Read the model definition and answer for the solid it produces. Units are mm, in the model's axes. A direction names the side the tool comes from. Give positions to 0.01 mm unless a question says otherwise; leave off trailing zeros. Order: outer loops, then holes, each group sorted by start corner. A loop starts at its lowest first (then second) coordinate and runs counter-clockwise, first axis right, second up. Notation, with made-up numbers: M -40,60.25 L -10,60.25 A13 ccw -10,67.25 Z; hole C -14,-29.5 d6. An arc over 180 degrees is marked long. Write item = value, one per line. Start each with the question number.
Autodesk Inventor part; units mm, degrees
ref_plane "YZ Plane" through (0, 0, 0) normal (1, 0, 0) x (0, 1, 0)
ref_plane "XZ Plane" through (0, 0, 0) normal (0, 1, 0) x (-1, 0, 0)
ref_plane "XY Plane" through (0, 0, 0) normal (0, 0, 1) x (1, 0, 0)
sketch "Sketch1" plane through (0, 0, 0) normal (0, 0, 1) x (1, 0, 0)
  circle A0 centre (0, 0) radius 35
  dimension "d0" = 70
extrude "Extrusion1" add sketch "Sketch1" along normal blind 50
sketch "Sketch4" plane through (0, 0, 50) normal (0, 0, 1) x (1, 0, 0)
  circle A0 centre (30, 0) radius 1.5
  dimension "d104" = 3
sketch "Sketch6" plane through (0, 0, 50) normal (0, 0, 1) x (1, 0, 0)
  circle A0 centre (-30, 0) radius 1.5
  point P0 (0, 0)
  dimension "d105" = 3
sketch "Sketch11" plane through (0, 0, 0) normal (0, 0, -1) x (-1, 0, 0)
  line L0 (13.8079, 12.25) -> (-13.8079, 12.25)
  line L1 (-18.25, 8.6641) -> (-18.25, -8.6641)
  line L2 (-13.8079, -12.25) -> (13.8079, -12.25)
  line L3 (18.25, -8.6641) -> (18.25, 8.6641)
  line L4 (17.3393, 10.3414) -> (14.8972, 11.9273)
  line L5 (17.3393, -10.3414) -> (14.8972, -11.9273)
  line L6 (-17.3393, 10.3414) -> (-14.8972, 11.9273)
  line L7 (-17.3393, -10.3414) -> (-14.8972, -11.9273)
  arc A0 (18.25, 8.6641) -> (17.3393, 10.3414) centre (16.25, 8.6641) ccw
  arc A1 (14.8972, 11.9273) -> (13.8079, 12.25) centre (13.8079, 10.25) ccw
  arc A2 (17.3393, -10.3414) -> (18.25, -8.6641) centre (16.25, -8.6641) ccw
  arc A3 (13.8079, -12.25) -> (14.8972, -11.9273) centre (13.8079, -10.25) ccw
  arc A4 (-14.8972, -11.9273) -> (-13.8079, -12.25) centre (-13.8079, -10.25) ccw
  arc A5 (-18.25, -8.6641) -> (-17.3393, -10.3414) centre (-16.25, -8.6641) ccw
  arc A6 (-17.3393, 10.3414) -> (-18.25, 8.6641) centre (-16.25, 8.6641) ccw
  arc A7 (-13.8079, 12.25) -> (-14.8972, 11.9273) centre (-13.8079, 10.25) ccw
  point P0 (18.25, 12.25)
  point P1 (-18.25, -12.25)
  point P2 (-18.25, 12.25)
  point P3 (18.25, -12.25)
  point P4 (18.25, 9.75)
  point P5 (18.25, -9.75)
  point P6 (-18.25, 9.75)
  point P7 (-18.25, -9.75)
  dimension "d73" = 36.5
  dimension "d74" = 24.5
  dimension "d75" = 2.5
  dimension "d76" = 57
  dimension "d77" = 2.5
  dimension "d78" = 57
  dimension "d79" = 2.5
  dimension "d80" = 57
  dimension "d81" = 2.5
  dimension "d82" = 57
  dimension "d83" = 2
extrude "Extrusion2" cut sketch "Sketch11" against normal blind 27.5
sketch "Sketch12" plane through (0, 0, 50) normal (0, 0, 1) x (1, 0, 0)
  line L0 (0, 0) -> (30, 0) construction
  line L1 (0, 0) -> (30, 0) construction
  arc A0 (-12.5, 21.6506) -> (-21.6506, 12.5) centre (0, 0) ccw
  arc A1 (-15, 25.9808) -> (-25.9808, 15) centre (0, 0) ccw
  arc A2 (25.9808, 15) -> (15, 25.9808) centre (0, 0) ccw
  arc A3 (21.6506, 12.5) -> (12.5, 21.6506) centre (0, 0) ccw
  arc A4 (15, -25.9808) -> (25.9808, -15) centre (0, 0) ccw
  arc A5 (12.5, -21.6506) -> (21.6506, -12.5) centre (0, 0) ccw
  arc A6 (-21.6506, -12.5) -> (-12.5, -21.6506) centre (0, 0) ccw
  arc A7 (-25.9808, -15) -> (-15, -25.9808) centre (0, 0) ccw
  line L2 (-21.6506, 12.5) -> (-25.9808, 15)
  line L3 (-12.5, 21.6506) -> (-15, 25.9808)
  line L4 (12.5, 21.6506) -> (15, 25.9808)
  line L5 (21.6506, 12.5) -> (25.9808, 15)
  line L6 (25.9808, -15) -> (21.6506, -12.5)
  line L7 (15, -25.9808) -> (12.5, -21.6506)
  line L8 (-12.5, -21.6506) -> (-15, -25.9808)
  line L9 (-21.6506, -12.5) -> (-25.9808, -15)
extrude "Extrusion3" cut sketch "Sketch12" against normal blind 10
fillet "Fillet3" radius 2 1 edges at (-35, 0, 0)
fillet "Fillet6" radius 1 16 edges at (12.5, 21.6506, 45) (21.6506, 12.5, 45) (25.9808, 15, 45) (15, 25.9808, 45) (-15, 25.9808, 45) (-12.5, 21.6506, 45) (-21.6506, 12.5, 45) (-25.9808, 15, 45) (-21.6506, -12.5, 45) (-25.9808, -15, 45) (-15, -25.9808, 45) (-12.5, -21.6506, 45) (12.5, -21.6506, 45) (15, -25.9808, 45) (25.9808, -15, 45) (21.6506, -12.5, 45)
sketch "Sketch15" plane through (0, 0, 27.5) normal (0, 0, -1) x (-1, 0, 0)
  circle A0 centre (-15.25, 0) radius 1.75
  circle A1 centre (-15.25, -6.5) radius 1.75
  circle A2 centre (-15.25, 6.5) radius 1.75
  point P0 (0, 0)
  dimension "d85" = 3.5
extrude "Extrusion6" add sketch "Sketch15" along normal blind 24
sketch "Sketch16" plane through (0, 0, 0) normal (0, 0, -1) x (-1, 0, 0)
  line L0 (-8, 23) -> (8, 23)
  line L1 (10, 21) -> (10, 20)
  line L2 (8, 18) -> (-8, 18)
  line L3 (-10, 20) -> (-10, 21)
  arc A0 (21.1538, 13.3235) -> (13.3235, 21.1538) centre (0, 0) ccw
  line L4 (8, -18) -> (-7.798, -18)
  line L5 (-9.798, -20) -> (-9.798, -21)
  line L6 (-7.798, -23) -> (8, -23)
  line L7 (10, -21) -> (10, -20)
  arc A1 (10, 21) -> (8, 23) centre (8, 21) ccw
  arc A2 (8, 18) -> (10, 20) centre (8, 20) ccw
  arc A3 (-10, 20) -> (-8, 18) centre (-8, 20) ccw
  arc A4 (-8, 23) -> (-10, 21) centre (-8, 21) ccw
  arc A5 (-7.798, -18) -> (-9.798, -20) centre (-7.798, -20) ccw
  arc A6 (10, -20) -> (8, -18) centre (8, -20) ccw
  arc A7 (8, -23) -> (10, -21) centre (8, -21) ccw
  arc A8 (-9.798, -21) -> (-7.798, -23) centre (-7.798, -21) ccw
  point P0 (0, 0)
  point P1 (10, 18)
  point P2 (10, 23)
  point P3 (-10, 18)
  point P4 (10, -18)
  point P5 (-9.798, -23)
  point P6 (-9.798, -18)
  dimension "d90" = 20
  dimension "d91" = 5
  dimension "d92" = 5
  dimension "d93" = 2
extrude "Extrusion7" cut sketch "Sketch16" against normal blind 10
extrude "Extrusion10" cut sketch "Sketch6" against normal through all
extrude "Extrusion11" cut sketch "Sketch4" against normal through all
equation "\"d78\" = d76"
properties part number "middle orbit" material "ABS Plastic"
1) For a pull along Y with two mould halves and no side action, classify faces 4 (the face through (13.751, -23.818, 45.07)), 5 (the face through (0, -14, 0)) as pulls with the +Y half, pulls with the -Y half, needs draft (parallel to the pull), parting line crosses it, or undercut.
2) Find section B-B on x = 0. Determine the outline of the cut face in (y, z), plus the area to 3 significant figures.
3) Find the intervals of material crossed by probe 1 along X at (y, z) = (19, 48.5); probe 2 along X at (y, z) = (23, 45.5); probe 3 along Y at (x, z) = (-21.5, 46), in increasing order. Write a range as [from, to].
4) For faces 1 (the face through (9.197, -18.57, 4.93)), 2 (the face through (-21.281, -21.146, 45.07)), 3 (the face through (28.5, 0.07, 25.35)), determine the directions among +Z, -Z, +X, -X, +Y, -Y from which every point of the face is accessible in a straight line to the end or side of a thin tool.
5) Find section A-A on y = 0. Determine the outline of the cut face in (x, z).
6) Each of these flat-tipped pins is pushed along its axis until it touches: P1, Ø5, axis at y = -2, z = 33.5, coming from the +X side; P2, Ø3, axis at x = 3.5, z = 6.5, coming from the -Y side; P3, Ø11, axis at x = 0, z = 5.5, coming from the -Y side; P4, Ø1.5, axis at y = 17.5, z = 28.5, coming from the +X side. Where does it stop, or does it pass through?
Numbers:
q1.face_4 = undercut
q1.face_5 = needs draft
q2.outline = M -35,2 A2 ccw -33,0 L -23,0 L -23,10 L -18,10 L -18,0 L -12.25,0 L -12.25,27.5 L 12.25,27.5 L 12.25,0 L 18,0 L 18,10 L 23,10 L 23,0 L 33,0 A2 ccw 35,2 L 35,50 L -35,50 Z
q2.area = 2,720 mm2
q3.probe_1 = [-29.39, -23.22], [-16.25, 16.25], [23.22, 29.39]
q3.probe_2 = [-26.38, -19.26], [-13.28, 13.28], [19.26, 26.38]
q3.probe_3 = [-27.62, -20.92], [-12.99, 12.99], [20.92, 27.62]
q4.face_1 = -Z
q4.face_2 = +Z
q4.face_3 = +Z, -Z
q5.outline = M -35,2 A2 ccw -33,0 L -31.5,0 L -31.5,50 L -35,50 Z; M -28.5,0 L -18.25,0 L -18.25,27.5 L 13.5,27.5 L 13.5,3.5 L 17,3.5 L 17,27.5 L 18.25,27.5 L 18.25,0 L 28.5,0 L 28.5,50 L -28.5,50 Z; M 31.5,0 L 33,0 A2 ccw 35,2 L 35,50 L 31.5,50 Z
q6.P1 = 35
q6.P2 = -34.94
q6.P3 = -35
q6.P4 = 30.73
